```python
from build123d import *

# Parameters (mm, degrees)
SKETCH1_W           = 23
SKETCH1_H           = 12.75
SKETCH1_R           = 1.65
BOSS_EXTRUDE1_DEPTH = 15
SKETCH2_R           = 1.65
CUT_EXTRUDE1_DEPTH  = 31.274783236
SKETCH3_R           = 5
CUT_EXTRUDE2_DEPTH  = 5
SKETCH4_OUTSIDE_W   = 31.054
SKETCH4_OUTSIDE_H   = 20.804
SKETCH4_OUTSIDE_W_2 = 22.5
SKETCH4_OUTSIDE_H_2 = 12.75
CUT_EXTRUDE3_DEPTH  = 31.274783236


with BuildPart() as part:
    # Sketch1 → Boss-Extrude1 (new body)
    with BuildSketch(Plane(origin=(0, 0, 0), x_dir=(1, 0, 0), z_dir=(0, 1, 0))):
        with Locations((11.5, 6.375)):
            Rectangle(SKETCH1_W, SKETCH1_H)
        with Locations(Location((4, 4, 0), (0, 0, 270))):
            Circle(SKETCH1_R, mode=Mode.SUBTRACT)
        with Locations(Location((19, 4, 0), (0, 0, 270))):
            Circle(SKETCH1_R, mode=Mode.SUBTRACT)
    extrude(amount=BOSS_EXTRUDE1_DEPTH)

    # Sketch2 → Cut-Extrude1 (cut, through all)
    with BuildSketch(Plane.XY):
        with Locations((11.5, 7.5)):
            Circle(SKETCH2_R)
    extrude(amount=-CUT_EXTRUDE1_DEPTH, mode=Mode.SUBTRACT)

    # Sketch3 → Cut-Extrude2 (cut)
    with BuildSketch(Plane.XY):
        with Locations((11.5, 7.5)):
            Circle(SKETCH3_R)
    extrude(amount=-CUT_EXTRUDE2_DEPTH, mode=Mode.SUBTRACT)

    # Sketch4 outside → Cut-Extrude3 (cut, through all)
    with BuildSketch(Plane(origin=(0, 15, 0), x_dir=(1, 0, 0), z_dir=(0, 1, 0))):
        with Locations((11.5, 6.375)):
            Rectangle(SKETCH4_OUTSIDE_W, SKETCH4_OUTSIDE_H)
        with Locations((11.5, 6.375)):
            Rectangle(SKETCH4_OUTSIDE_W_2, SKETCH4_OUTSIDE_H_2, mode=Mode.SUBTRACT)
    extrude(amount=-CUT_EXTRUDE3_DEPTH, mode=Mode.SUBTRACT)


solid = part.part
```
Could you check a few things on this model? Use its own coordinates, in mm. A direction names the side the tool comes from. Round coordinates to 2 decimals unless told otherwise and drop trailing zeros. Order: outer loops, then holes, each group sorted by start corner. A loop starts at its lowest first (then second) coordinate and runs counter-clockwise, first axis right, second up. Notation, with made-up numbers: M -25.5,73 L 24.5,73 A16 ccw 24.5,81 Z; hole C -4.75,50.5 d5. An arc over 180 degrees is marked long. One line per question, with ' | ' between items. Start each with the question number.
(1) Please list where these lines run through material, in increasing order: line 1 along X through (y, z) = (6.75, -4); line 2 along X through (y, z) = (9.5, -2.5); line 3 along X through (y, z) = (5.5, -0.5).
(2) For P1, Ø3, axis at x = 12, y = 5.5, coming from the +Z side; P2, Ø2, axis at x = 4, z = -4, coming from the -Y side, each with a flat end and sliding along its axis, tell me the tip position at first contact or that it passes through.
(3) Suppose I cut it at A-A on y = 7.5. List the corners of the cut face in (x, z) for me.
(4) Thinking about a two-plate mould opening in Y: for faces 1 (the face through (11, 0, -6)), 2 (the face through (10, 9, -5)), 3 (the face through (6, 7, 0)), which applies, +Y half, -Y half, draft (parallel to the pull), parting line (faces both ways), or undercut?
(5) Suppose I cut it at D-D on y = 10.5. List the corners of the cut face in (x, z) for me, then the cut area to 3 significant figures.
(6) Suppose I cut it at C-C on z = -4. List the corners of the cut face in (x, y) for me.
(7) Suppose I cut it at B-B on x = 19. List the corners of the cut face in (y, z) for me.
(8) For faces 4 (the face through (22.75, 8, -6)), 5 (the face through (16.27, 9, -2.46)), which set-ups out of +Z, -Z, +X, -X, +Y, -Y let a thin tool reach every point of the face, with its end or its side?
Geometry results:
1) line 1: 0.25 to 2.35, 5.65 to 6.56, 16.44 to 17.35, 20.65 to 22.75 | line 2: 0.25 to 3.31, 4.69 to 6.92, 16.08 to 18.31, 19.69 to 22.75 | line 3: 0.25 to 6.92, 16.08 to 22.75
2) P1: z = -5 | P2: through
3) outline: M 0.25,-12.75 L 9.85,-12.75 L 9.85,-5 L 6.5,-5 L 6.5,0 L 0.25,0 Z; M 13.15,-12.75 L 22.75,-12.75 L 22.75,0 L 16.5,0 L 16.5,-5 L 13.15,-5 Z; hole C 4,-4 d3.3; hole C 19,-4 d3.3
4) face 1: -Y half | face 2: undercut | face 3: draft
5) outline: M 0.25,-12.75 L 22.75,-12.75 L 22.75,0 L 15.5,0 L 15.5,-5 L 7.5,-5 L 7.5,0 L 0.25,0 Z; hole C 4,-4 d3.3; hole C 19,-4 d3.3 | area: 230 mm²
6) outline: M 0.25,0 L 2.35,0 L 2.35,15 L 0.25,15 Z; M 5.65,0 L 17.35,0 L 17.35,15 L 5.65,15 Z; M 20.65,0 L 22.75,0 L 22.75,15 L 20.65,15 Z; hole C 11.5,7.5 d10
7) outline: M 0,-12.75 L 15,-12.75 L 15,-5.65 L 0,-5.65 Z; M 0,-2.35 L 15,-2.35 L 15,0 L 0,0 Z
8) face 4: +Z, -Z, +X, +Y, -Y | face 5: +Z
